Verification items for this drawing (mm, ordinates from the low corner). Coordinates: 2 decimals unless noted, no trailing zeros. Order: outer loops, then holes, each group sorted by start corner. A loop starts at its lowest first (then second) coordinate and runs counter-clockwise, first axis right, second up. Notation, with made-up numbers: (35.5, 13.25) -> (79.5, 13.25) arc R27 ccw to (79.5, 47.25) -> close; hole circle Ø5 at (7.25, -19.5). An arc over 180 degrees is marked (long way). Write item = value, one per line. Start each with the question number.
1. Thickness scan on line 1 along Y through (x, z) = (13.5, 2.45) (3 decimals); line 2 along Y through (x, z) = (139.7, 0.75) (3 decimals); line 3 along Y through (x, z) = (131, 1.65) (3 decimals). Record the ranges inside material, lowest first. Write a range as from..to.
2. Cross-section at A-A on y = 101.6. Record the cut outline in (x, z) (3 decimals).
3. Cross-section at C-C on z = 0.5. Give the number of separate pieces and of enclosed holes in the cut face, plus the area to 4 significant figures.
4. Cross-section at B-B on x = 149. Record the cut outline in (y, z) (3 decimals), plus the area to 3 significant figures.
5. Go/stop test with flat-tipped pins: P1, Ø1.6, axis at x = 19.5, z = 1, coming from the +Y side (3 decimals); P2, Ø7.5, axis at x = 50.8, y = 101.6, coming from the -Z side. Record where each tip stops, or that it passes through.
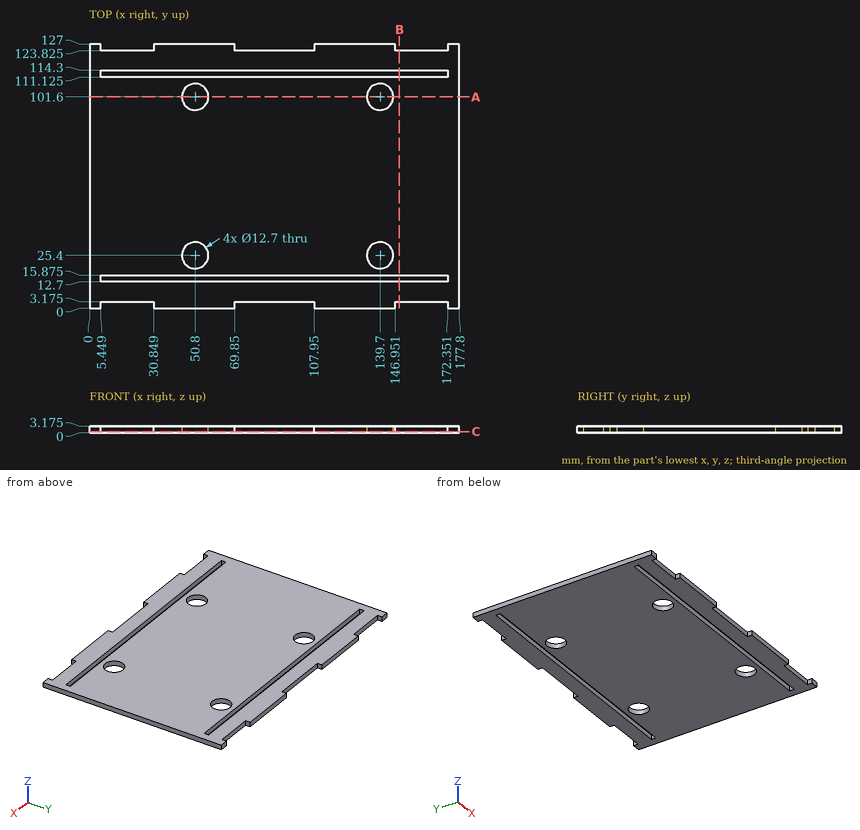
Worked out:
q1.line_1 = 3.175..12.7, 15.875..111.125, 114.3..123.825
q1.line_2 = 0..12.7, 15.875..19.05, 31.75..95.25, 107.95..111.125, 114.3..127
q1.line_3 = 0..12.7, 15.875..111.125, 114.3..127
q2.outline = (0, 0) -> (44.45, 0) -> (44.45, 3.175) -> (0, 3.175) -> close; (57.15, 0) -> (133.35, 0) -> (133.35, 3.175) -> (57.15, 3.175) -> close; (146.05, 0) -> (177.8, 0) -> (177.8, 3.175) -> (146.05, 3.175) -> close
q3.separate_pieces = 1
q3.enclosed_holes = 6
q3.area = 20,450 mm²
q4.outline = (3.175, 0) -> (12.7, 0) -> (12.7, 3.175) -> (3.175, 3.175) -> close; (15.875, 0) -> (111.125, 0) -> (111.125, 3.175) -> (15.875, 3.175) -> close; (114.3, 0) -> (123.825, 0) -> (123.825, 3.175) -> (114.3, 3.175) -> close
q4.area = 363 mm²
q5.P1 = 123.825
q5.P2 = through
